For this review, take the finished solid that the model builds, in its own axes (mm). Coordinates: 2 decimals unless noted, no trailing zeros. Loops run counter-clockwise (first coordinate to the right, second up) from the corner with the lowest first, then second, coordinate; pieces in that order, holes last.
1. Clearance check with flat-ended pins moving along their axes: P1, Ø3, axis at x = 12.5, z = 4.5, coming from the +Y side; P2, Ø0.5, axis at y = 0.5, z = -9, coming from the +X side; P3, Ø0.5, axis at y = 0.5, z = -8, coming from the -X side; P4, Ø0.5, axis at x = 4.5, y = 0.5, coming from the -Z side. State where each tip first meets the part, or that it passes through.
2. Take a section at A-A, the plane x = 8.25. State the section outline as (y, z) points.
3. Take a section at D-D, the plane z = -2.75. State the section outline as (x, y) points.
4. Take a section at B-B, the plane z = -7.5. State the section outline as (x, y) points, then the cut area to 3 significant figures.
5. To check wall thickness, follow probe 1 along X at (y, z) = (0.35, -7); probe 2 along Z at (x, y) = (4, 0.75); probe 3 along X at (y, z) = (0.7, -5.75). State the ranges of each line that lie inside material, in increasing order.
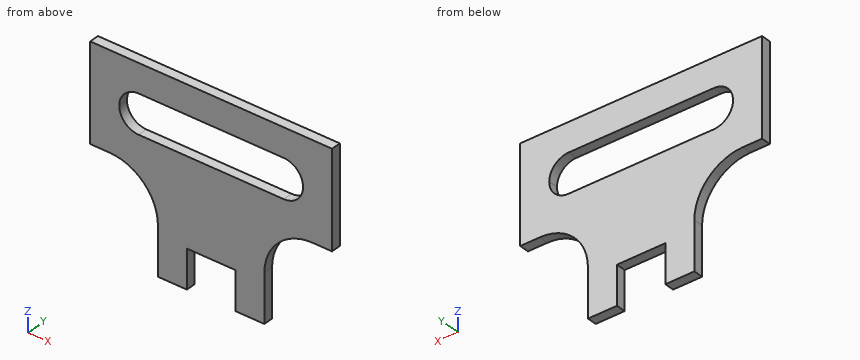
```python
from build123d import *

# Parameters (mm, degrees)
BOSS_EXTRUDE1_DEPTH = 1


with BuildPart() as part:
    # Sketch1 → Boss-Extrude1 (new body)
    with BuildSketch(Plane(origin=(0, 0, 0), x_dir=(1, 0, 0), z_dir=(0, 1, 0))):
        with BuildLine():
            Line((-0.811022124, 5.668679597), (-0.811022124, 10.668679597))
            Line((-0.811022124, 10.668679597), (2.188977876, 10.668679597))
            Line((2.188977876, 10.668679597), (2.188977876, 6.668679597))
            Line((2.188977876, 6.668679597), (7.188977876, 6.668679597))
            Line((7.188977876, 6.668679597), (7.188977876, 10.668679597))
            Line((7.188977876, 10.668679597), (10.188977876, 10.668679597))
            Line((10.188977876, 10.668679597), (10.188977876, 5.668679597))
            ThreePointArc((10.188977876, 5.668679597), (11.65344397, 2.133145691), (15.188977876, 0.668679597))
            Line((15.188977876, 0.668679597), (17.188977876, 0.668679597))
            Line((17.188977876, 0.668679597), (17.188977876, -9.331320403))
            Line((17.188977876, -9.331320403), (-7.811022124, -9.331320403))
            Line((-7.811022124, -9.331320403), (-7.811022124, 0.668679597))
            Line((-7.811022124, 0.668679597), (-5.811022124, 0.668679597))
            ThreePointArc((-5.811022124, 0.668679597), (-2.275488218, 2.133145691), (-0.811022124, 5.668679597))
        make_face()
        with BuildLine():
            Line((-2.811022124, -2.331320403), (12.188977876, -2.331320403))
            ThreePointArc((12.188977876, -2.331320403), (13.603191438, -2.917106841), (14.188977876, -4.331320403))
            Line((14.188977876, -4.331320403), (14.188977876, -4.346932121))
            ThreePointArc((14.188977876, -4.346932121), (13.603191438, -5.761145684), (12.188977876, -6.346932121))
            Line((12.188977876, -6.346932121), (-2.811022124, -6.346932121))
            ThreePointArc((-2.811022124, -6.346932121), (-4.225235686, -5.761145684), (-4.811022124, -4.346932121))
            Line((-4.811022124, -4.346932121), (-4.811022124, -4.331320403))
            ThreePointArc((-4.811022124, -4.331320403), (-4.225235686, -2.917106841), (-2.811022124, -2.331320403))
        make_face(mode=Mode.SUBTRACT)
    extrude(amount=BOSS_EXTRUDE1_DEPTH)


solid = part.part
```
Results list:
1. P1: passes through
1. P2: stops at x = 10.19
1. P3: stops at x = -0.81
1. P4: stops at z = -6.67
2. outline: (0, -10.67) - (1, -10.67) - (1, 2.33) - (0, 2.33) - close; (0, 6.35) - (1, 6.35) - (1, 9.33) - (0, 9.33) - close
3. outline: (-1.75, 0) - (11.13, 0) - (11.13, 1) - (-1.75, 1) - close
4. outline: (-0.81, 0) - (2.19, 0) - (2.19, 1) - (-0.81, 1) - close; (7.19, 0) - (10.19, 0) - (10.19, 1) - (7.19, 1) - close
4. area: 6.00 mm2
5. probe 1: x = -0.81 to 2.19, 7.19 to 10.19
5. probe 2: z = -6.67 to 2.33, 6.35 to 9.33
5. probe 3: x = -0.81 to 10.19
